Here's the drawing with two shaded views (mm, measured from the low corner). I have some questions. A direction names the side the tool comes from. Round coordinates to 2 decimals unless told otherwise and drop trailing zeros. Order: outer loops, then holes, each group sorted by start corner. A loop starts at its lowest first (then second) coordinate and runs counter-clockwise, first axis right, second up.
Q1. If we section it at A-A (z = 47.8): Please give me the cut outline in (x, y), plus the area to 3 significant figures.
Q2. If we section it at D-D (x = 56): Please give me the cut outline in (y, z), plus the area to 3 significant figures.
Q3. If I drill on line 1 (Y direction, x = 2.75, z = 47.8); line 2 (Z direction, x = 7.5, y = 2.5); line 3 (X direction, y = 7.5, z = 59), over which ranges is the centre line in solid material (lowest first)?
Q4. For the marked faces 1 and 2, which set-ups out of +Z, -Z, +X, -X, +Y, -Y let a thin tool reach every point of the face, with its end or its side?
Q5. Will these pins go through, and if not, where does the flat tip stop? P1, Ø6, axis at x = 34.5, y = 12, coming from the -Z side; P2, Ø6, axis at y = 12.5, z = 29.5, coming from the +X side.
Q6. If we section it at C-C (y = 5.25): Please give me the cut outline in (x, z), plus the area to 3 significant figures.
Q7. If we section it at B-B (y = 8.65): Please give me the cut outline in (x, z).
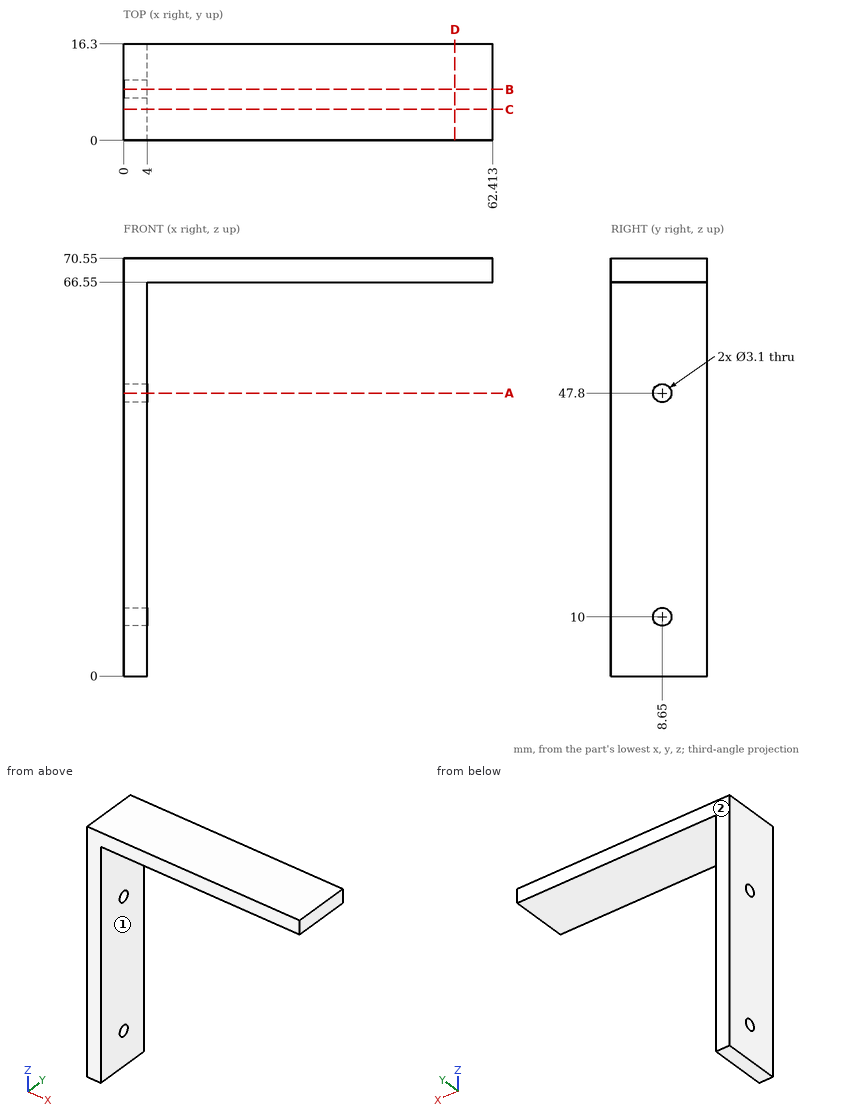
Solution:
1. outline: (0, 0) - (4, 0) - (4, 7.1) - (0, 7.1) - close; (0, 10.2) - (4, 10.2) - (4, 16.3) - (0, 16.3) - close
1. area: 52.8 mm2
2. outline: (0, 66.55) - (16.3, 66.55) - (16.3, 70.55) - (0, 70.55) - close
2. area: 65.2 mm2
3. line 1: y = 0 to 7.1, 10.2 to 16.3
3. line 2: z = 66.55 to 70.55
3. line 3: x = 0 to 4
4. face 1: -Z, +X, +Y, -Y
4. face 2: +Z, -Z, +X, -X, +Y
5. P1: stops at z = 66.55
5. P2: stops at x = 4
6. outline: (0, 0) - (4, 0) - (4, 66.55) - (62.41, 66.55) - (62.41, 70.55) - (0, 70.55) - close
6. area: 516 mm2
7. outline: (0, 0) - (4, 0) - (4, 8.45) - (0, 8.45) - close; (0, 11.55) - (4, 11.55) - (4, 46.25) - (0, 46.25) - close; (0, 49.35) - (4, 49.35) - (4, 66.55) - (62.41, 66.55) - (62.41, 70.55) - (0, 70.55) - close
